Drawing for the job (mm, zero at the part's lowest x, y, z). Give positions to 0.01 mm unless a question says otherwise; leave off trailing zeros. Loops run counter-clockwise (first coordinate to the right, second up) from the corner with the lowest first, then second, coordinate; pieces in that order, holes last. Notation, with made-up numbers: (-38.5, 71) -> (-23.5, 71) arc R25 cw to (-23.5, 97) -> close; hole circle Ø5 at (59, -2). An arc over 180 degrees is marked (long way). Use CSV: the item, a comma, the result in double quotes. Start each with the question number.
(1) Cut at A-A on z = 60.5. Write the cut outline in (x, y).
(2) Drill centre lines: probe 1 along X at (y, z) = (1.3, 38.5); probe 2 along X at (y, z) = (5.7, 24.5); probe 3 along Z at (x, y) = (13.5, 5.55). Where is each one in solid material? Low to high.
(3) Flat gauge pins, fed straight in: pin 1 (5 mm diameter, centred on x = 157, z = 36, fed in from -Y); pin 2 (1.5 mm diameter, centred on y = 4, z = 34, fed in from -X); pin 3 (3 mm diameter, centred on y = 2, z = 38, fed in from -X); pin 4 (1.3 mm diameter, centred on y = 2, z = 34, fed in from +X). Where does each tip first touch, or does it go through?
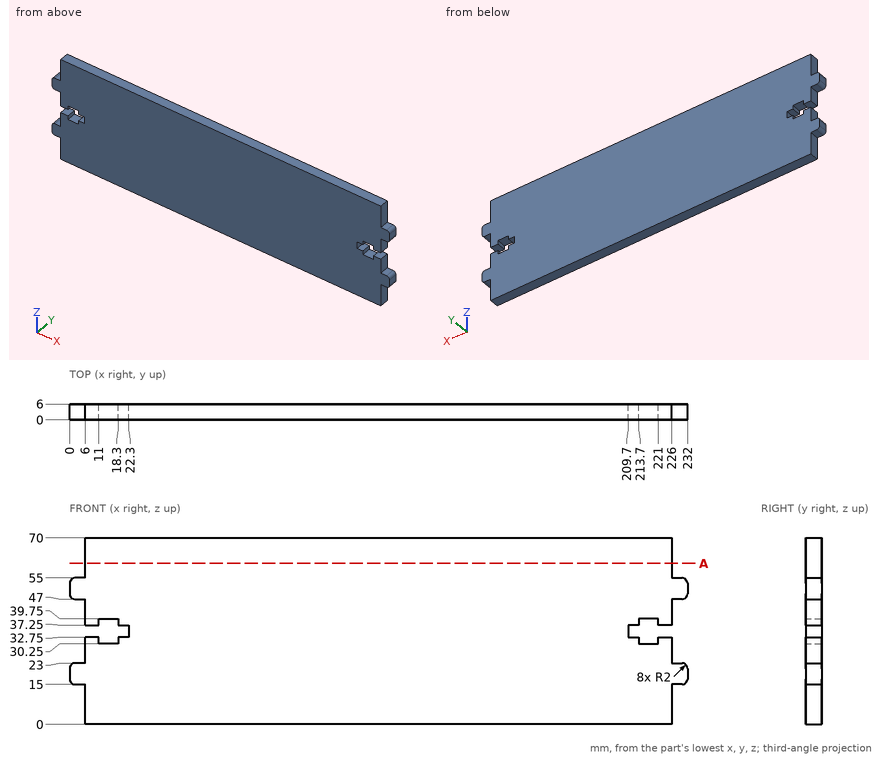
Check result:
1,outline,"(6, 0) -> (226, 0) -> (226, 6) -> (6, 6) -> close"
2,probe 1,"6 to 11, 18.3 to 213.7, 221 to 226"
2,probe 2,"6 to 226"
2,probe 3,"0 to 30.25, 39.75 to 70"
3,pin 1,"y = 0"
3,pin 2,"x = 22.3"
3,pin 3,"x = 6"
3,pin 4,"x = 209.7"
